from build123d import *

# Parameters (mm, degrees)
SKETCH_1_W      = 220
SKETCH_1_H      = 195
SKETCH_1_W_2    = 200
SKETCH_1_H_2    = 8
SKETCH_1_H_3    = 12
SKETCH_1_H_4    = 16
SKETCH_1_H_5    = 24
SKETCH_1_H_6    = 44
EXTRUDE_1_DEPTH = 6


with BuildPart() as part:
    # Эскиз1 → Бобышка-Вытянуть1 (new body)
    with BuildSketch(Plane.XY):
        with Locations((0, 26.5)):
            Rectangle(SKETCH_1_W, SKETCH_1_H)
        with Locations((0, 110)):
            Rectangle(SKETCH_1_W_2, SKETCH_1_H_2, mode=Mode.SUBTRACT)
        with Locations((0, 97)):
            Rectangle(SKETCH_1_W_2, SKETCH_1_H_2, mode=Mode.SUBTRACT)
        with Locations((0, 82)):
            Rectangle(SKETCH_1_W_2, SKETCH_1_H_3, mode=Mode.SUBTRACT)
        with Locations((0, 65)):
            Rectangle(SKETCH_1_W_2, SKETCH_1_H_3, mode=Mode.SUBTRACT)
        with Locations((0, 46)):
            Rectangle(SKETCH_1_W_2, SKETCH_1_H_4, mode=Mode.SUBTRACT)
        with Locations((0, 25)):
            Rectangle(SKETCH_1_W_2, SKETCH_1_H_4, mode=Mode.SUBTRACT)
        Rectangle(SKETCH_1_W_2, SKETCH_1_H_5, mode=Mode.SUBTRACT)
        with Locations((0, -39)):
            Rectangle(SKETCH_1_W_2, SKETCH_1_H_6, mode=Mode.SUBTRACT)
    extrude(amount=EXTRUDE_1_DEPTH)


solid = part.part
Geometry: final body of the model. Coordinates: model frame, mm. A direction names the side the tool comes from. Give positions to 0.01 mm unless a question says otherwise; leave off trailing zeros. Write each loop counter-clockwise with the first axis right and the second up, starting at its lowest first coordinate (ties: lowest second). Pieces come first, ordered by that corner, then holes. Notation, with made-up numbers: M 1,38.25 L 53,38.25 A20 cw 53,59.25 Z; hole C -13.75,70.25 d9. An arc over 180 degrees is marked long. Answer in a Markdown table with one row per item. Add a question column.
(1) Mould query, pull axis Y, two halves, no side actions, for faces 1 (the flat face through (-1.5, 71.2, 6)), 2 (the flat face through (-1, 59, 3)). Classes: +Y half, -Y half, draft (parallel to the pull), parting line (faces both ways), or undercut.
(2) Reachability of faces 3 (the flat face through (-110, 25, 3)), 4 (the flat face through (100, 46, 3)) from +Z, -Z, +X, -X, +Y, -Y: full face, straight path, thin tool, end or side. Return the list, or none.
(3) Ray query, line 1 (X direction, y = -31.5, z = 0.75). Return the intervals inside material, ascending.
(4) Section A-A on y = 45.5. Return loops of the section in (x, z).
(5) Section B-B on z = 1.9. State how many separate pieces and enclosed holes the cut face has, and give its area (3 significant figures).
Result set:
| question | item | result |
|---|---|---|
| 1 | face 1 | draft |
| 1 | face 2 | undercut |
| 2 | face 3 | +Z, -Z, -X, +Y, -Y |
| 2 | face 4 | +Z, -Z |
| 3 | line 1 | x = -110 to -100, 100 to 110 |
| 4 | outline | M -110,0 L -100,0 L -100,6 L -110,6 Z; M 100,0 L 110,0 L 110,6 L 100,6 Z |
| 5 | separate pieces | 1 |
| 5 | enclosed holes | 8 |
| 5 | area | 14,900 mm^2 |
